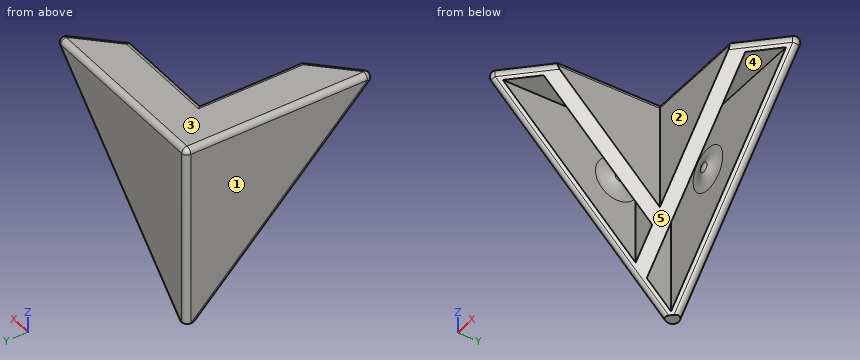
```python
from build123d import *

# Parameters (mm, degrees)
F1_DEPTH  = 28.575
F3_R      = 38.1
F4_DEPTH  = 32.9965678842
F6_W      = 26.9748
F6_H      = 3.429
F6_W_2    = 3.429
F6_H_2    = 21.971
F7_DEPTH  = 26.9758
F14_R     = 0.762
F15_W     = 1.8396307345
F15_H     = 3.0181135691
F16_DEPTH = 26.4941772846


# Not quite as in the source:
# - a fillet or chamfer that OpenCascade refuses, or shapes differently, is made with other operations: its cross-section is extruded or revolved along the edge and cut away or added
# - a pattern or mirror of a feature is missing from the dataset's text; its kind, count and spacing are read off the source's solid


with BuildPart() as f1:
    # F0 (on Top) → F1 (new body)
    with BuildSketch(Plane.XY):
        Polygon((0, -21.971), (0, 0), (21.971, 0), (21.971, 6.604), (-6.604, 6.604), (-6.604, -21.971), align=None)
    extrude(amount=-F1_DEPTH)

    # F3 (on 3pt) → F4 (cut, through all)
    with BuildSketch(Plane(origin=(5.1223333333, -5.1223333333, -5.1223333333), x_dir=(0.4082482905, 0.8164965809, -0.4082482905), z_dir=(0.5773502692, -0.5773502692, -0.5773502692))):
        Circle(F3_R)
    extrude(amount=F4_DEPTH, mode=Mode.SUBTRACT)

    # F6 (on offset) → F7 (cut, through all)
    with BuildSketch(Plane.XY.offset(-1.6002)):
        with Locations((8.4836, 3.2893)):
            Rectangle(F6_W, F6_H)
        with Locations((-3.2893, -10.9855)):
            Rectangle(F6_W_2, F6_H_2)
    extrude(amount=-F7_DEPTH, mode=Mode.SUBTRACT)

    # F9 (on offset) → F10 (revolve)
    with BuildSketch(Plane.YZ.offset(2.6162)):
        with BuildLine():
            ThreePointArc((4.2418, -9.2202), (4.4469151823, -9.9607308906), (5.0038, -10.4902))
            Line((5.0038, -10.4902), (5.0038, -9.2202))
            Line((5.0038, -9.2202), (4.2418, -9.2202))
        make_face()
    f10 = revolve(axis=Axis((2.6162, 4.6228, -9.2202), (0, -1, 0)))

    # F10_copies: F10 across plane
    add(f10.mirror(Plane(origin=(0, 0, 0), x_dir=(0.7071067796, -0.7071067828, 0), z_dir=(-0.7071067828, -0.7071067796, 0))))

    # F13: fillet of radius 5.08 on 3 edges, made by hand

    # F13_s1 → F13_t2 (revolve)
    with BuildSketch(Plane.YZ.offset(2.6162)):
        with BuildLine():
            ThreePointArc((5.0038, -12.278765023), (4.853123865, -11.0506908258), (4.4100337662, -9.8954676025))
            ThreePointArc((4.4100337662, -9.8954676025), (4.662543942, -10.2371346569), (5.0038, -10.4902))
            Line((5.0038, -10.4902), (5.0038, -12.278765023))
        make_face()
    revolve(axis=Axis((2.6162, 5.0038, -9.2202), (0, -1, 0)))

    # F13_s3 → F13_t4 (revolve)
    with BuildSketch(Plane.XZ.offset(2.6161999777)):
        with BuildLine():
            ThreePointArc((-5.0038, -12.2787650011), (-4.8531238674, -11.0506908133), (-4.4100337753, -9.8954675976))
            ThreePointArc((-4.4100337753, -9.8954675976), (-4.6625439517, -10.237134655), (-5.0038000116, -10.4902))
            Line((-5.0038000116, -10.4902), (-5.0038, -12.2787650011))
        make_face()
    revolve(axis=Axis((-5.0038000116, -2.6161999777, -9.2202), (-1, 4.4e-09, 0)))

    # F14
    f14_edges = [f1.edges().sort_by_distance(p)[0] for p in [
        (7.6835, 6.604, 0),
        (-6.604, 6.604, -14.2875),
        (7.6835, 6.604, -14.2875),
        (-6.604, -7.6835, 0),
        (-6.604, -7.6835, -14.2875),
        (18.669, 3.302, 0),
        (7.6835, 0, 0),
        (0, -7.6835, 0),
        (-3.302, -18.669, 0),
    ]]
    fillet(f14_edges, radius=F14_R)

    # F15 (on face) → F16 (cut, through all)
    with BuildSketch(Plane(origin=(-6.604, 0, 0), x_dir=(0, -1, 0), z_dir=(-1, 0, 0))):
        with Locations((-5.6841846327, -27.2402340692)):
            Rectangle(F15_W, F15_H)
    extrude(amount=-F16_DEPTH, mode=Mode.SUBTRACT)


solid = f1.part
```
Design review of the part built by this model. Coordinates are the model's own, in mm. Face numbers are marked on the shaded views. A direction names the side the tool comes from. Coordinates: 2 decimals unless noted, no trailing zeros.
1) To check wall thickness, follow L1, parallel to X at y = -11.5, z = -2.5; L2, parallel to Y at x = -4.5, z = -13.5; L3, parallel to Z at x = 3, y = 2. State the ranges of each line that lie inside material, in increasing order.
2) Machinability: for the marked faces 1 and 2, which of the approach directions +Z, -Z, +X, -X, +Y, -Y give a long, thin tool a straight path to every point of the face, cutting with its end or side? Answer none if there is none.
3) Mouldability with a two-part tool opening along Y and no side actions: class the marked faces 3, 4 and 5 as +Y half, -Y half, draft (parallel to the pull), parting line (faces both ways), or undercut.
4) Insertion check: pin 1 (8 mm diameter, centred on y = -7.5, z = -5, fed in from +X); pin 2 (1 mm diameter, centred on x = -3.5, y = -11, fed in from -Z); pin 3 (4.5 mm diameter, centred on x = 8.5, z = -8, fed in from -Y); pin 4 (12 mm diameter, centred on x = 16.5, z = -4.5, fed in from +Y). Each pin has a flat end and moves straight along its axis. Give the tip position at first contact, or say it passes through.
Check result:
1. L1: x = -6.6 to -5, -1.57 to 0
1. L2: y = 0 to 1.57, 5 to 6.6
1. L3: z = -1.6 to 0
2. face 1: +Z, -Z, -X, +Y, -Y
2. face 2: +Z, -Z, +X, -Y
3. face 3: draft
3. face 4: undercut
3. face 5: -Y half
4. pin 1: stops at x = 0
4. pin 2: stops at z = -1.6
4. pin 3: stops at y = 0
4. pin 4: stops at y = 6.6
